For this review, take the finished solid that the model builds, in its own axes (mm). Face numbers are marked on the shaded views. Round coordinates to 2 decimals unless told otherwise and drop trailing zeros. Loops run counter-clockwise (first coordinate to the right, second up) from the corner with the lowest first, then second, coordinate; pieces in that order, holes last. Notation, with made-up numbers: M -4.75,-10 L 39.25,-10 A23 ccw 39.25,29 Z; hole C 34.25,-2 d4. An arc over 180 degrees is marked long. Write item = value, one per line. Start each with the question number.
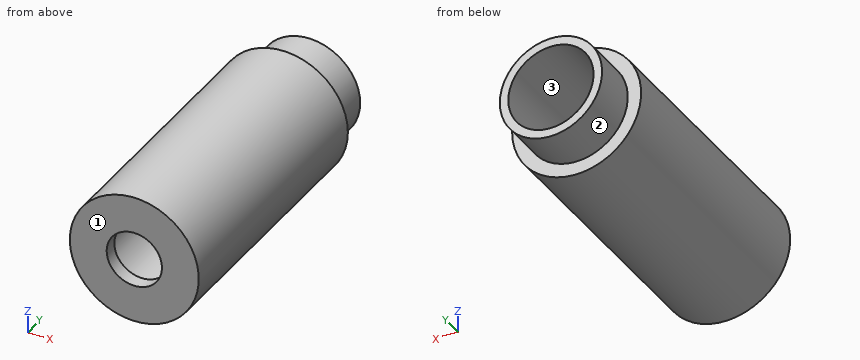
Autodesk Inventor part; units mm, degrees
ref_plane "YZ Plane" through (0, 0, 0) normal (1, 0, 0) x (0, 1, 0)
ref_plane "XZ Plane" through (0, 0, 0) normal (0, 1, 0) x (-1, 0, 0)
ref_plane "XY Plane" through (0, 0, 0) normal (0, 0, 1) x (1, 0, 0)
sketch "Sketch1" plane through (0, 0, 0) normal (0, 1, 0) x (-1, 0, 0)
  circle A0 centre (0, 0) radius 140
  circle A1 centre (0, 0) radius 60
  dimension "d0" = 280
  dimension "d1" = 120
extrude "Extrusion1" add sketch "Sketch1" along normal blind 30
sketch "Sketch3" plane through (0, 30, 0) normal (0, 1, 0) x (1, 0, 0)
  circle A0 centre (0, 0) radius 92.5
  circle A1 centre (0, 0) radius 140
  dimension "d12" = 185
  dimension "d18" = 280
extrude "Extrusion3" add sketch "Sketch3" along normal blind 550
sketch "Sketch4" plane through (0, 580, 0) normal (0, 1, 0) x (1, 0, 0)
  circle A0 centre (0, 0) radius 60
  circle A1 centre (0, 0) radius 111
  circle A2 centre (0, 0) radius 92.5
  dimension "d15" = 222
  dimension "d19" = 185
extrude "Extrusion4" add sketch "Sketch4" along normal blind 100 contours A1
properties part number "taoa"
(1) For pin 1 Ø12 at (y, z) = (126.5, -36.5) entering from +X; pin 2 Ø3 at (y, z) = (199.5, 5) entering from +X; pin 3 Ø8 at (y, z) = (150.5, -42) entering from +X, all flat-tipped, find the tip position at first contact; note any pin that passes through.
(2) Wall thickness on L1, parallel to Z at x = 0, y = 10.75; L2, parallel to Z at x = -1, y = 183.5; L3, parallel to X at y = 289, z = 0: over which ranges is each line inside the solid? List them lowest first.
(3) Draft analysis for pull direction X (two halves, no side actions). For the marked faces 1, 2 and 3, state which applies: +X half, -X half, draft (parallel to the pull), parting line (faces both ways), or undercut.
(4) Add section C-C on y = 175. Write out the cut boundary in (x, z).
(5) Add section A-A on z = -27.5. Write out the cut boundary in (x, y), and give its area (3 significant figures).
Answer sheet:
q1.pin_1 = 136.64
q1.pin_2 = 139.96
q1.pin_3 = 134.74
q2.L1 = -140 to -60, 60 to 140
q2.L2 = -140 to -92.49, 92.49 to 140
q2.L3 = -140 to -92.5, 92.5 to 140
q3.face_1 = draft
q3.face_2 = parting line
q3.face_3 = undercut
q4.outline = C 0,0 d280; hole C 0,0 d185
q5.outline = M -137.27,0 L -53.33,0 L -53.33,30 L -88.32,30 L -88.32,680 L -107.54,680 L -107.54,580 L -137.27,580 Z; M 53.33,0 L 137.27,0 L 137.27,580 L 107.54,580 L 107.54,680 L 88.32,680 L 88.32,30 L 53.33,30 Z
q5.area = 62,700 mm²
